Verification items for the finished model (mm, model axes). Face numbers are marked on the shaded views. Round coordinates to 2 decimals unless told otherwise and drop trailing zeros. Order: outer loops, then holes, each group sorted by start corner. A loop starts at its lowest first (then second) coordinate and runs counter-clockwise, first axis right, second up. Notation, with made-up numbers: (45.5, 7) -> (75.5, 7) arc R16 ccw to (75.5, 29) -> close; hole circle Ø7 at (-37.75, 29.25). An arc over 180 degrees is marked (long way). Put each result on its own line as item: value.
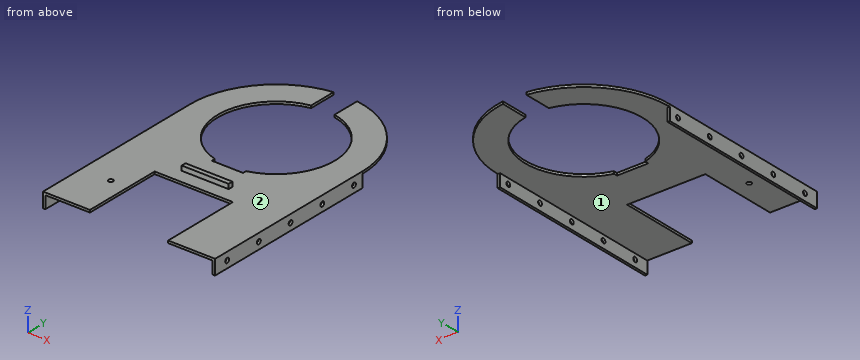
Autodesk Inventor part; units mm, degrees
ref_plane "YZ Plane" through (0, 0, 0) normal (1, 0, 0) x (0, 1, 0)
ref_plane "XZ Plane" through (0, 0, 0) normal (0, 1, 0) x (-1, 0, 0)
ref_plane "XY Plane" through (0, 0, 0) normal (0, 0, 1) x (1, 0, 0)
sketch "Skizze1" plane through (0, 0, 0) normal (0, 0, 1) x (1, 0, 0)
  line L0 (-25, 0) -> (-25, 51)
  line L1 (-25, 51) -> (25, 51)
  line L2 (25, 51) -> (25, 0)
  line L3 (25, 0) -> (55, 0)
  line L4 (55, 0) -> (55, 116)
  arc A0 (55, 116) -> (-55, 116) centre (0, 116) ccw
  line L5 (-55, 116) -> (-55, 0)
  line L6 (-55, 0) -> (-25, 0)
  point P0 (0, 0)
  point P1 (0, 51)
  point P2 (-40, 0)
  dimension "d0" = 25
  dimension "d1" = 51
  dimension "d2" = 116
  dimension "d3" = 55
extrude "Extrusion1" add sketch "Skizze1" along normal mid plane 1.5
sketch "Skizze2" plane through (0, 0, 0.75) normal (0, 0, 1) x (1, 0, 0)
  line L0 (-25, 51) -> (25, 51)
  line L1 (25, 51) -> (25, 0)
  line L2 (25, 0) -> (55, 0)
  line L3 (55, 0) -> (55, 116)
  arc A0 (55, 116) -> (-55, 116) centre (0, 116) ccw
  line L4 (-55, 116) -> (-55, 0)
  line L5 (-55, 0) -> (-25, 0)
  line L6 (-25, 0) -> (-25, 51)
  circle A1 centre (0, 116) radius 37.5
  point P0 (0, 0)
  dimension "d6" = 75
extrude "Extrusion2" cut sketch "Skizze2" against normal up to surface (1.5 mm away) contours A1
sketch "Skizze3" plane through (0, 0, 0.75) normal (0, 0, 1) x (1, 0, 0)
  arc A0 (55, 116) -> (-55, 116) centre (0, 116) ccw
  circle A1 centre (0, 116) radius 37.5
  line L0 (-7.5, 152.7423) -> (-7.5, 170.4862)
  line L1 (7.5, 152.7423) -> (7.5, 170.4862)
  line L2 (0, 116) -> (0, 135.7591) construction
  line L3 (-10, 79.8579) -> (-10, 77.5)
  line L4 (-10, 77.5) -> (10, 77.5)
  line L5 (10, 77.5) -> (10, 79.8579)
  point P0 (0, 0)
  dimension "d9" = 15
  dimension "d12" = 20
  dimension "d13" = 1
extrude "Extrusion3" cut sketch "Skizze3" against normal up to surface (1.5 mm away) contours L1 A1 L0 A0
extrude "Extrusion4" cut sketch "Skizze3" against normal up to surface (1.5 mm away) contours A1 L5 L4 L3
sketch "Skizze5" plane through (0, 0, 0.75) normal (0, 0, 1) x (1, 0, 0)
  line L0 (-15, 63) -> (15, 63)
  line L1 (15, 63) -> (15, 60)
  line L2 (15, 60) -> (-15, 60)
  line L3 (-15, 60) -> (-15, 63)
  point P0 (0, 0)
  point P1 (0, 60)
  dimension "d16" = 3
  dimension "d17" = 30
  dimension "d18" = 60
extrude "Extrusion5" add sketch "Skizze5" along normal blind 3
sketch "Sketch9" plane through (55, 0, 0.75) normal (1, 0, 0) x (0, 0, -1)
  line L0 (1.5, 116) -> (1.5, 0)
  line L1 (0, 0) -> (0, 116)
  line L2 (1.5, 116) -> (0, 116)
  line L3 (1.5, 0) -> (0, 0)
  line L4 (9.5, 0) -> (9.5, 116)
  line L5 (1.5, 116) -> (1.5, 0)
  line L6 (9.5, 116) -> (0, 116)
  line L7 (0, 0) -> (9.5, 0)
  point P0 (0.75, 0)
  dimension "d39" = 8
extrude "Extrusion7" add sketch "Sketch9" against normal blind 1.5
sketch "Sketch8" plane through (55, 0, 0.75) normal (1, 0, 0) x (0, 0, -1)
  line L0 (0, 0) -> (0, 116)
  point P0 (0.75, 0)
  point P1 (5, 109.5)
  point P2 (5, 84.5)
  point P3 (5, 59.5)
  point P4 (5, 34.5)
  point P5 (5, 9.5)
  dimension "d26" = 25
  dimension "d27" = 25
  dimension "d28" = 25
  dimension "d29" = 25
  dimension "d30" = 5
hole "Hole1" at (55, 109.5, -4.25) at (55, 84.5, -4.25) at (55, 59.5, -4.25) at (55, 34.5, -4.25) at (55, 9.5, -4.25) direction (-1, 0, 0) diameter 3 depth 1.5
mirror "Mirror1" about plane through (0, 0, 0) normal (1, 0, 0) of "Hole1", "Extrusion7"
sketch "Sketch10" plane through (0, 0, 0.75) normal (0, 0, 1) x (1, 0, 0)
  line L0 (-55, 0) -> (-25, 0)
  line L1 (-55, 116) -> (-55, 0)
  point P0 (0, 0)
  point P1 (-36, 30)
  dimension "d42" = 30
  dimension "d43" = 19
hole "Hole2" at (-36, 30, 0.75) direction (0, 0, -1) diameter 3 depth 1.5
properties part number "1 part 06"
Item 1: Gauge pin test, flat ends, axial feed: pin 1 Ø4 at (y, z) = (9.5, -4.25) entering from -X; pin 2 Ø1.2 at (x, z) = (-3, 0) entering from +Y; pin 3 Ø6 at (y, z) = (149.5, -3.5) entering from -X; pin 4 Ø5 at (x, y) = (26.5, 148) entering from -Z. Record the tip position at first contact, or that the pin passes through.
Check sheet entries:
pin 1: stops at x = -55
pin 2: stops at y = 77.5
pin 3: stops at x = -44.52
pin 4: stops at z = -0.75
Item 2: Section check D-D on y = 118. Record the boundary of the cut face in (x, z), then the cut area to 3 significant figures.
Check sheet entries:
outline: (-54.96, -0.75) -> (-37.45, -0.75) -> (-37.45, 0.75) -> (-54.96, 0.75) -> close; (37.45, -0.75) -> (54.96, -0.75) -> (54.96, 0.75) -> (37.45, 0.75) -> close
area: 52.6 mm^2
Item 3: Section check B-B on x = 4. Record the boundary of the cut face in (y, z).
Check sheet entries:
outline: (51, -0.75) -> (77.5, -0.75) -> (77.5, 0.75) -> (63, 0.75) -> (63, 3.75) -> (60, 3.75) -> (60, 0.75) -> (51, 0.75) -> close
Item 4: Section check C-C on x = 23. Record the boundary of the cut face in (y, z), then the cut area to 3 significant figures.
Check sheet entries:
outline: (51, -0.75) -> (86.38, -0.75) -> (86.38, 0.75) -> (51, 0.75) -> close; (145.62, -0.75) -> (165.96, -0.75) -> (165.96, 0.75) -> (145.62, 0.75) -> close
area: 83.6 mm^2
Item 5: Section check A-A on y = 22. Record the boundary of the cut face in (x, z), then the cut area to 3 significant figures.
Check sheet entries:
outline: (-55, -8.75) -> (-53.5, -8.75) -> (-53.5, -0.75) -> (-25, -0.75) -> (-25, 0.75) -> (-55, 0.75) -> close; (25, -0.75) -> (53.5, -0.75) -> (53.5, -8.75) -> (55, -8.75) -> (55, 0.75) -> (25, 0.75) -> close
area: 114 mm^2
Item 6: Material ranges on L1, parallel to Y at x = 54.4, z = -4.25; L2, parallel to X at y = 30, z = 0.15; L3, parallel to Z at x = -53.85, y = 9.5, recorded low to high. Write a range as [from, to].
Check sheet entries:
L1: y = [0, 8], [11, 33], [36, 58], [61, 83], [86, 108], [111, 116]
L2: x = [-55, -37.5], [-34.5, -25], [25, 55]
L3: z = [-8.75, -5.75], [-2.75, 0.75]
Item 7: Release check for a two-part mould opening along X. For the marked faces 1 and 2 record: +X half, -X half, draft (parallel to the pull), parting line (faces both ways), or undercut.
Check sheet entries:
face 1: undercut
face 2: draft
